The figure shows three views and two pictorial views of one solid part (mm, origin at its lowest corner). Answer the questions. A direction names the side the tool comes from. Give positions to 0.01 mm unless a question says otherwise; leave off trailing zeros. Loops run counter-clockwise (first coordinate to the right, second up) from the corner with the lowest first, then second, coordinate; pieces in that order, holes last. Notation, with made-up numbers: (65.5, -1.75) -> (81.5, -1.75) arc R24 ccw to (81.5, 18.25) -> close; hole circle Ø9 at (52, -34). An arc over 180 degrees is marked (long way). Answer as CSV lines item,"result". Start each with the question number.
1. Find section C-C, the plane z = 19.05. Give the vertices of the cut face in (x, y).
2. Find the intervals of material crossed by line 1 along X through (y, z) = (133.5, 31.5); line 2 along Y through (x, z) = (37, 19), in increasing order.
3. Find section B-B, the plane y = 82.55. Give the vertices of the cut face in (x, z) (1 decimal).
4. A tool of negligible diameter and unlimited length cuts with its end or side. For the marked faces 5 and 6, from which of +Z, -Z, +X, -X, +Y, -Y can it reach the whole face along a straight path? Write none if from no direction.
5. Find section D-D, the plane x = 10.5. Give the vertices of the cut face in (y, z).
6. Determine the mould class of the marked faces 1, 2, 3 and 4 for opening direction Z: +Z half, -Z half, draft (parallel to the pull), parting line (faces both ways), or undercut.
7. Find section A-A, the plane z = 7.5. Give the vertices of the cut face in (x, y).
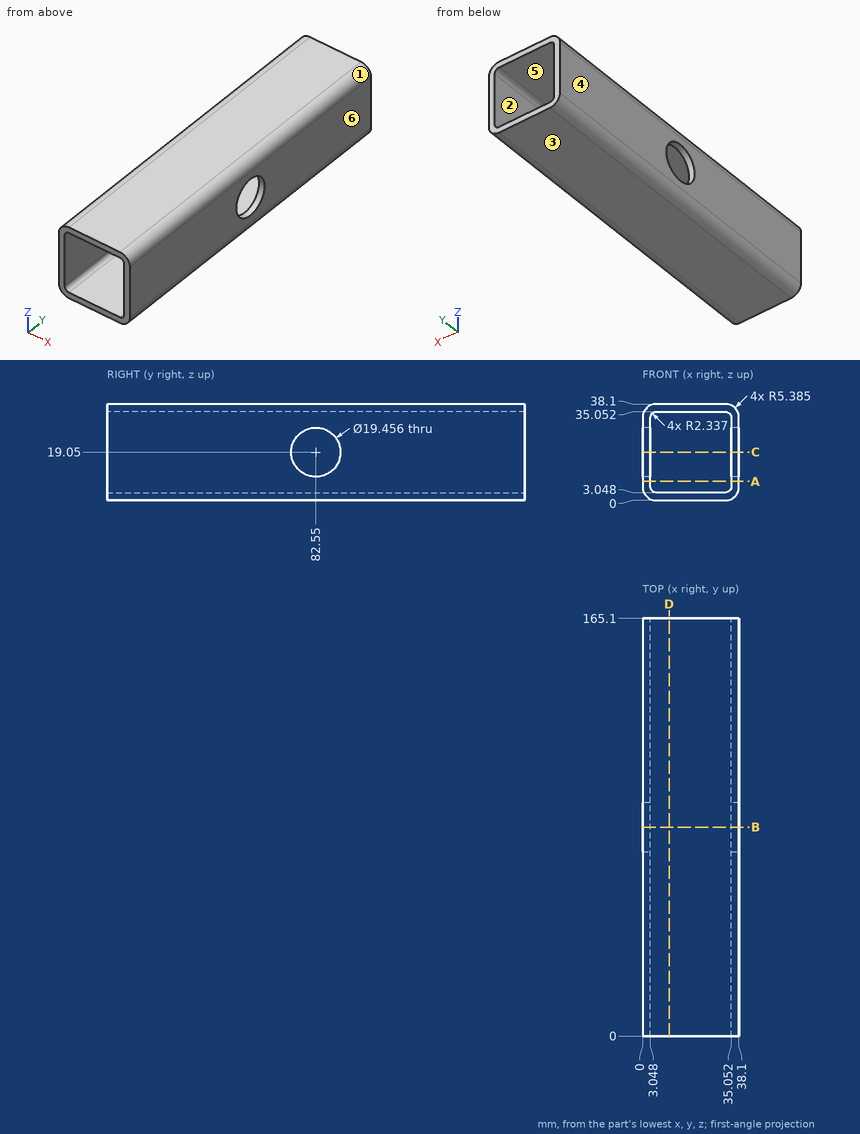
Resolved:
1,outline,"(0, 0) -> (3.05, 0) -> (3.05, 72.82) -> (0, 72.82) -> close; (0, 92.28) -> (3.05, 92.28) -> (3.05, 165.1) -> (0, 165.1) -> close; (35.05, 0) -> (38.1, 0) -> (38.1, 72.82) -> (35.05, 72.82) -> close; (35.05, 92.28) -> (38.1, 92.28) -> (38.1, 165.1) -> (35.05, 165.1) -> close"
2,line 1,"x = 0 to 3.05, 35.05 to 38.1"
2,line 2,"y = 0 to 72.82, 92.28 to 165.1"
3,outline,"(0, 5.4) arc R5.4 ccw to (5.4, 0) -> (32.7, 0) arc R5.4 ccw to (38.1, 5.4) -> (38.1, 9.3) -> (35.1, 9.3) -> (35.1, 5.4) arc R2.3 cw to (32.7, 3) -> (5.4, 3) arc R2.3 cw to (3, 5.4) -> (3, 9.3) -> (0, 9.3) -> close; (0, 28.8) -> (3, 28.8) -> (3, 32.7) arc R2.3 cw to (5.4, 35.1) -> (32.7, 35.1) arc R2.3 cw to (35.1, 32.7) -> (35.1, 28.8) -> (38.1, 28.8) -> (38.1, 32.7) arc R5.4 ccw to (32.7, 38.1) -> (5.4, 38.1) arc R5.4 ccw to (0, 32.7) -> close"
4,face 5,"+Y, -Y"
4,face 6,"+Z, -Z, +X, +Y, -Y"
5,outline,"(0, 0) -> (165.1, 0) -> (165.1, 3.05) -> (0, 3.05) -> close; (0, 35.05) -> (165.1, 35.05) -> (165.1, 38.1) -> (0, 38.1) -> close"
6,face 1,"+Z half"
6,face 2,"undercut"
6,face 3,"-Z half"
6,face 4,"draft"
7,outline,"(0, 0) -> (3.05, 0) -> (3.05, 165.1) -> (0, 165.1) -> close; (35.05, 0) -> (38.1, 0) -> (38.1, 165.1) -> (35.05, 165.1) -> close"
